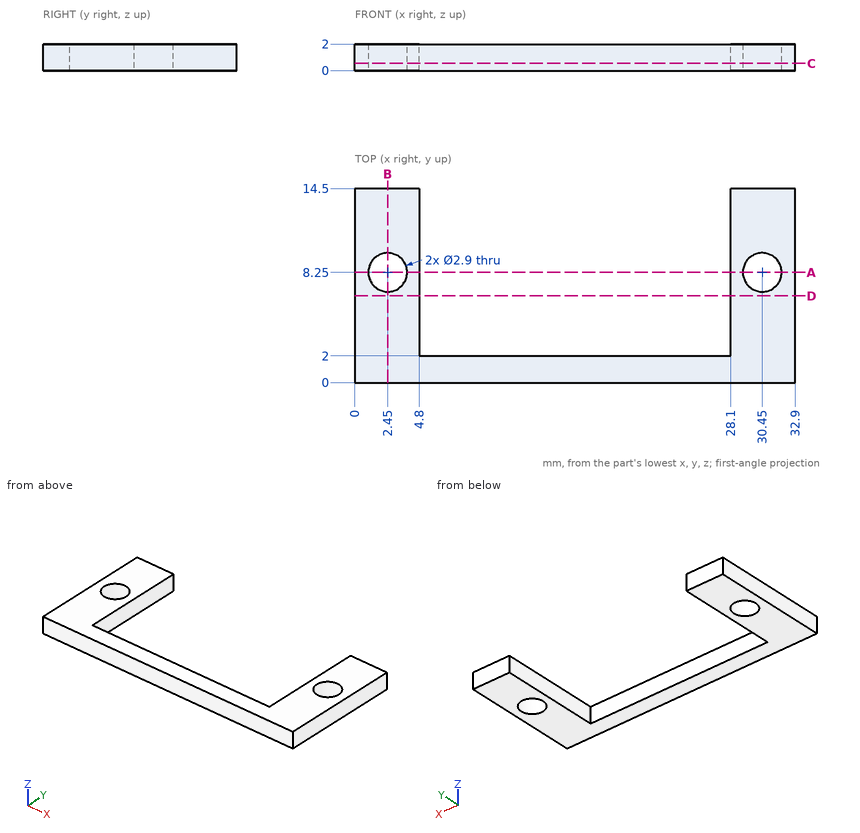
Input: dimensioned drawing with shaded views. Units: mm. Origin: part minimum x, y, z. Round coordinates to 2 decimals unless told otherwise and drop trailing zeros. Loops run counter-clockwise (first coordinate to the right, second up) from the corner with the lowest first, then second, coordinate; pieces in that order, holes last. Notation, with made-up numbers: M 54.25,70.25 L 87.25,70.25 A25 cw 87.25,84.25 Z; hole C 3.5,60.25 d11. An arc over 180 degrees is marked long. Return JSON: item names as keys, results as strings. Group by question number.
1. Section query D-D on y = 6.5. Output: boundary loops of the cut face in (x, z).
2. Section query B-B on x = 2.45. Output: boundary loops of the cut face in (y, z), and give its area (3 significant figures).
3. Material intervals for line 1 along X through (y, z) = (6.25, 1.05); line 2 along Y through (x, z) = (30.45, 0.9); line 3 along Y through (x, z) = (11, 0.65), sorted ascending. Write a range as from..to.
4. Pin query (flat end, axial travel): pin 1 (2.5 mm diameter, centred on x = 2.45, y = 8.25, fed in from -Z); pin 2 (0.6 mm diameter, centred on x = 11.5, z = 1, fed in from +Y). Return the tip coordinate at first contact, or that it passes through.
5. Section query C-C on z = 0.55. Output: boundary loops of the cut face in (x, y), and give its area (3 significant figures).
6. Section query A-A on y = 8.25. Output: boundary loops of the cut face in (x, z), and give its area (3 significant figures).
Checks:
{
 "1": {"outline": "M 0,0 L 4.8,0 L 4.8,2 L 0,2 Z; M 28.1,0 L 32.9,0 L 32.9,2 L 28.1,2 Z"},
 "2": {"outline": "M 0,0 L 6.8,0 L 6.8,2 L 0,2 Z; M 9.7,0 L 14.5,0 L 14.5,2 L 9.7,2 Z", "area": "23.2 mm²"},
 "3": {"line 1": "x = 0..4.8, 28.1..32.9", "line 2": "y = 0..6.8, 9.7..14.5", "line 3": "y = 0..2"},
 "4": {"pin 1": "passes through", "pin 2": "stops at y = 2"},
 "5": {"outline": "M 0,0 L 32.9,0 L 32.9,14.5 L 28.1,14.5 L 28.1,2 L 4.8,2 L 4.8,14.5 L 0,14.5 Z; hole C 2.45,8.25 d2.9; hole C 30.45,8.25 d2.9", "area": "173 mm²"},
 "6": {"outline": "M 0,0 L 1,0 L 1,2 L 0,2 Z; M 3.9,0 L 4.8,0 L 4.8,2 L 3.9,2 Z; M 28.1,0 L 29,0 L 29,2 L 28.1,2 Z; M 31.9,0 L 32.9,0 L 32.9,2 L 31.9,2 Z", "area": "7.60 mm²"}
}
